from build123d import *

# Parameters (mm, degrees)
SKETCH_1_W                   = 160
SKETCH_1_H                   = 60
EXTRUDE_1_DEPTH              = 60
SKETCH_2_W                   = 30
SKETCH_2_H                   = 50
CUT_EXTRUDE_1_DEPTH          = 114.648581161
SKETCH_3_W                   = 30
SKETCH_3_H                   = 50
CUT_EXTRUDE_2_DEPTH          = 114.648581161
SKETCH_4_W                   = 69.99999994
SKETCH_4_H                   = 6
CUT_EXTRUDE_3_DEPTH          = 114.648581161
EXTRUDE_2_DEPTH              = 10
EXTRUDE_3_DEPTH              = 10
SKETCH_7_W                   = 70.000000048
SKETCH_7_H                   = 30
CUT_EXTRUDE_4_DEPTH          = 15
HOLE_WIZARD_M52_1_D          = 60
HOLE_WIZARD_12_0_12_1_D      = 12
HOLE_WIZARD_12_0_12_1_DEPTH  = 10
HOLE_WIZARD_12_0_12_2_D      = 12
HOLE_WIZARD_12_0_12_2_DEPTH  = 10
HOLE_WIZARD_M8_1_D           = 9
HOLE_WIZARD_M8_1_DEPTH       = 10
HOLE_WIZARD_M8_1_CBORE_D     = 18
HOLE_WIZARD_M8_1_CBORE_DEPTH = 0.5
FILLET_1_R                   = 15
FILLET_2_R                   = 2


with BuildPart() as part:
    # 草图1 → 凸台-拉伸1 (new body)
    with BuildSketch(Plane(origin=(0, 54, 0), x_dir=(1, 0, 0), z_dir=(0, 1, 0))):
        Rectangle(SKETCH_1_W, SKETCH_1_H)
    extrude(amount=-EXTRUDE_1_DEPTH)

    # 草图2 → 切除-拉伸1 (cut, through all)
    with BuildSketch(Plane(origin=(0, 0, -30), x_dir=(-1, 0, 0), z_dir=(0, 0, -1))):
        with Locations((-65, 29)):
            Rectangle(SKETCH_2_W, SKETCH_2_H)
    extrude(amount=-CUT_EXTRUDE_1_DEPTH, mode=Mode.SUBTRACT)

    # 草图3 → 切除-拉伸2 (cut, through all)
    with BuildSketch(Plane(origin=(0, 0, -30), x_dir=(-1, 0, 0), z_dir=(0, 0, -1))):
        with Locations((65, 29)):
            Rectangle(SKETCH_3_W, SKETCH_3_H)
    extrude(amount=-CUT_EXTRUDE_2_DEPTH, mode=Mode.SUBTRACT)

    # 草图4 → 切除-拉伸3 (cut, through all)
    with BuildSketch(Plane(origin=(0, 0, -30), x_dir=(-1, 0, 0), z_dir=(0, 0, -1))):
        with Locations((0, -3)):
            Rectangle(SKETCH_4_W, SKETCH_4_H)
    extrude(amount=-CUT_EXTRUDE_3_DEPTH, mode=Mode.SUBTRACT)

    # 草图5 → 凸台-拉伸2 (add)
    with BuildSketch(Plane(origin=(0, 54, 0), x_dir=(1, 0, 0), z_dir=(0, 1, 0))):
        with BuildLine():
            Line((-50, -15), (-50, 15))
            Line((-50, 15), (-70, 15))
            ThreePointArc((-70, 15), (-85, 0), (-70, -15))
            Line((-70, -15), (-50, -15))
        make_face()
    extrude(amount=-EXTRUDE_2_DEPTH)

    # 草图6 → 凸台-拉伸3 (add)
    with BuildSketch(Plane(origin=(0, 54, 0), x_dir=(1, 0, 0), z_dir=(0, 1, 0))):
        with BuildLine():
            Line((50, 15), (50, -15))
            Line((50, -15), (70, -15))
            ThreePointArc((70, -15), (85, 0), (70, 15))
            Line((70, 15), (50, 15))
        make_face()
    extrude(amount=-EXTRUDE_3_DEPTH)

    # 草图7 → 切除-拉伸4 (cut)
    with BuildSketch(Plane(origin=(0, 54, 0), x_dir=(-1, 0, 0), z_dir=(0, 1, 0))):
        Rectangle(SKETCH_7_W, SKETCH_7_H)
    extrude(amount=-CUT_EXTRUDE_4_DEPTH, mode=Mode.SUBTRACT)

    # M52 间隙孔1 (through all)
    with Locations(Plane(origin=(0, 0, -30), x_dir=(-1, 0, 0), z_dir=(0, 0, -1))):
        with Locations((0, 54)):
            Hole(HOLE_WIZARD_M52_1_D / 2)

    # Ø12.0 (12) 直径孔1
    with Locations(Plane(origin=(0, 44, 0), x_dir=(-1, 0, 0), z_dir=(0, -1, 0))):
        with Locations((-70, 0)):
            Hole(HOLE_WIZARD_12_0_12_1_D / 2, depth=HOLE_WIZARD_12_0_12_1_DEPTH)

    # Ø12.0 (12) 直径孔2
    with Locations(Plane(origin=(0, 54, 0), x_dir=(1, 0, 0), z_dir=(0, 1, 0))):
        with Locations((-70, 0)):
            Hole(HOLE_WIZARD_12_0_12_2_D / 2, depth=HOLE_WIZARD_12_0_12_2_DEPTH)

    # M8 六角头螺栓的柱形沉头孔1
    with Locations(Plane(origin=(0, 4, 0), x_dir=(1, 0, 0), z_dir=(0, 1, 0))):
        with Locations((-65, -15), (-65, 15), (65, 15), (65, -15)):
            CounterBoreHole(HOLE_WIZARD_M8_1_D / 2, HOLE_WIZARD_M8_1_CBORE_D / 2, HOLE_WIZARD_M8_1_CBORE_DEPTH, depth=HOLE_WIZARD_M8_1_DEPTH)

    # 圆角1
    fillet_1_edges = [part.edges().sort_by_distance(p)[0] for p in [
        (80, -1, 30),
        (-80, -1, 30),
        (-80, -1, -30),
        (80, -1, -30),
    ]]
    fillet(fillet_1_edges, radius=FILLET_1_R)

    # 圆角2
    fillet_2_edges = [part.edges().sort_by_distance(p)[0] for p in [
        (80, 4, 0),
        (57.5, 4, -30),
        (57.5, 4, 30),
        (75.606601718, 4, 25.606601718),
        (75.606601718, 4, -25.606601718),
        (-80, 4, 0),
        (-75.606601718, 4, 25.606601718),
        (-75.606601718, 4, -25.606601718),
        (50, 4, 0),
        (50, 29, 30),
        (50, 29, -30),
        (-57.5, 4, 30),
        (-50, 29, 30),
        (-50, 4, 0),
        (-50, 29, -30),
        (-57.5, 4, -30),
        (34.99999997, 0, 0),
        (-34.99999997, 0, 0),
        (-60, 44, 15),
        (-50, 49, 15),
        (-85, 44, 0),
        (-60, 44, -15),
        (-50, 44, 0),
        (-50, 49, -15),
        (60, 44, -15),
        (50, 49, -15),
        (85, 44, 0),
        (60, 44, 15),
        (50, 44, 0),
        (50, 49, 15),
    ]]
    fillet(fillet_2_edges, radius=FILLET_2_R)


solid = part.part
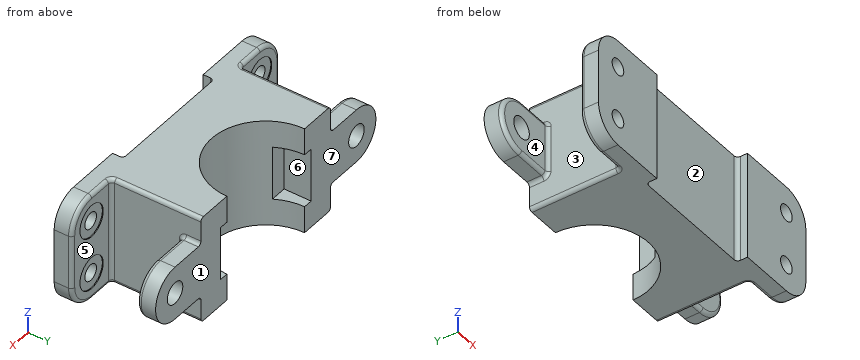
Check sheet for the modelled part. Datum: model origin and axes. Units: mm. Face numbers are marked on the shaded views. A direction names the side the tool comes from. Round coordinates to 2 decimals unless told otherwise and drop trailing zeros. Order: outer loops, then holes, each group sorted by start corner. A loop starts at its lowest first (then second) coordinate and runs counter-clockwise, first axis right, second up. Notation, with made-up numbers: M -25,86.5 L -2,86.5 A27 cw -2,103.5 Z; hole C 14.5,56.25 d2. An arc over 180 degrees is marked long. One line per item, written item: value. Start each with the question number.
1. Section check A-A on y = 36. Enter the section's corners in (x, z).
2. Scan lines: line 1 along Z through (x, y) = (65, 0); line 2 along Y through (x, z) = (-57.5, -6.5); line 3 along Z through (x, y) = (-65, 3.7). Record each from-to range of solid material in increasing order.
3. Release check for a two-part mould opening along X. For the marked faces 1, 2 and 3 record: released by +X, released by -X, zero draft, split by the parting line, or undercut.
4. Section check C-C on y = 14. Enter the section's corners in (x, z), and give its area (3 significant figures).
5. Access from +Z, -Z, +X, -X, +Y, -Y to the whole of each face (thin tool, end or side, straight path). Record for the marked faces 4, 5, 6 and 7.
6. Section check B-B on z = 0. Give the number of separate pieces and of enclosed holes in the cut face, and give its area (3 significant figures).
7. Gauge pin test, flat ends, axial feed: P1, Ø3, axis at y = -4, z = -2.5, coming from the +X side; P2, Ø3, axis at x = -5.5, z = 0.5, coming from the -Y side; P3, Ø1, axis at y = 24, z = -5, coming from the +X side. Record the tip position at first contact, or that the pin passes through.
Results found:
1. outline: M -50,-28 A2 ccw -48,-30 L -24,-30 L -24,30 L -48,30 A2 ccw -50,28 Z; M 24,-30 L 48,-30 A2 ccw 50,-28 L 50,28 A2 ccw 48,30 L 24,30 Z
2. line 1: -30 to -19.5, -10.5 to 10.5, 19.5 to 30
2. line 2: -6 to 4, 44 to 54
2. line 3: -29.05 to -24, -6 to 6, 24 to 29.05
3. face 1: zero draft
3. face 2: undercut
3. face 3: released by -X
4. outline: M -50,-28 A2 ccw -48,-30 L 48,-30 A2 ccw 50,-28 L 50,28 A2 ccw 48,30 L -48,30 A2 ccw -50,28 Z
4. area: 6,000 mm^2
5. face 4: +Z, -Z, -X
5. face 5: +Z, -Z, +X
5. face 6: +Y
5. face 7: +Z, -Z, +X, -X, +Y
6. separate pieces: 3
6. enclosed holes: 0
6. area: 5,040 mm^2
7. P1: x = 80
7. P2: y = 0
7. P3: x = 50
